from build123d import *

# Parameters (mm, degrees)
SKETCH1_W           = 7.2
SKETCH1_H           = 10.8
SKETCH1_R           = 1.75
BOSS_EXTRUDE3_DEPTH = 5
SKETCH2_W           = 50
SKETCH2_H           = 20
BOSS_EXTRUDE4_DEPTH = 5


with BuildPart() as part:
    # Sketch1 → Boss-Extrude3 (new body)
    with BuildSketch(Plane.XY):
        with Locations((10.9, 2.5)):
            Rectangle(SKETCH1_W, SKETCH1_H)
        Polygon((-20, 22.5), (-30, 11.319660113), (-30, -7.5), (-20, -22.5), (-4, -22.5), (6, -7.5), (30, -7.5), (30, 12.5), (6, 12.5), (-4, 22.5), align=None)
        with Locations((-17, -17.5)):
            Circle(SKETCH1_R, mode=Mode.SUBTRACT)
        with Locations((-7, -17.5)):
            Circle(SKETCH1_R, mode=Mode.SUBTRACT)
        with Locations((-25, 2.5)):
            Circle(SKETCH1_R, mode=Mode.SUBTRACT)
        Polygon((-3.5, 7.9), (7.3, 7.9), (14.5, 7.9), (14.5, -2.9), (7.3, -2.9), (-3.5, -2.9), align=None, mode=Mode.SUBTRACT)
    extrude(amount=BOSS_EXTRUDE3_DEPTH)

    # Sketch2 → Boss-Extrude4 (add)
    with BuildSketch(Plane(origin=(0, 0, 0), x_dir=(-1, 0, 0), z_dir=(0, 0, -1))):
        with Locations((-5, 2.5)):
            Rectangle(SKETCH2_W, SKETCH2_H)
    extrude(amount=-BOSS_EXTRUDE4_DEPTH)


solid = part.part
Source: CAD feature listing. Evaluate the final solid. Frame: model axes, mm. A direction names the side the tool comes from. Give positions to 0.01 mm unless a question says otherwise; leave off trailing zeros. Write each loop counter-clockwise with the first axis right and the second up, starting at its lowest first coordinate (ties: lowest second). Pieces come first, ordered by that corner, then holes. Notation, with made-up numbers: M 74,88.25 L 84,88.25 A11 ccw 84,97.25 Z; hole C 73,65 d3. An arc over 180 degrees is marked long. Return JSON: item names as keys, results as strings. Group by question number.
1) Cut plane C-C, the plane x = -25. Output: boundary loops of the cut face in (y, z).
2) Set-up query: faces 1 (the face through (-7, 0, 0)), 2 (the face through (18, -7.5, 2)), 3 (the face through (18, 12.5, 2)). Return all of +Z, -Z, +X, -X, +Y, -Y with unobstructed straight access to the full face (end or side cutting, diameter ignored); none if empty.
3) Cut plane D-D, the plane y = -17.5. Output: boundary loops of the cut face in (x, z).
4) Cut plane A-A, the plane y = 2.5. Output: boundary loops of the cut face in (x, z).
5) Cut plane B-B, the plane z = 2.1. Output: boundary loops of the cut face in (x, y), plus the area to 3 significant figures.
6) Material intervals for line 1 along Y through (x, z) = (-17, 2.15); line 2 along Y through (x, z) = (-8.5, 1.35); line 3 along X through (y, z) = (1, 1.4), sorted ascending. Write a range as [from, to].
7) Pull-direction query (Y, two-part tool) for faces 4 (the face through (-26.75, 2.58, 2.46)), 5 (the face through (-30, 2, 2)), 6 (the face through (-24.93, 16.99, 2.46)); classes: pulls with the +Y half, pulls with the -Y half, needs draft (parallel to the pull), parting line crosses it, or undercut.
8) Pin query (flat end, axial travel): P1, Ø3, axis at x = -17, y = -17.5, coming from the +Z side; P2, Ø2.5, axis at x = 20.5, z = 3, coming from the -Y side. Return the tip coordinate at first contact, or that it passes through.
Recorded:
{
 "1": {"outline": "M -15,0 L 0.75,0 L 0.75,5 L -15,5 Z; M 4.25,0 L 16.91,0 L 16.91,5 L 4.25,5 Z"},
 "2": {"face 1": "-Z, +X, -X, +Y, -Y", "face 2": "+Z, -Z, +X, -Y", "face 3": "+Z, -Z, +X, +Y"},
 "3": {"outline": "M -23.33,0 L -18.75,0 L -18.75,5 L -23.33,5 Z; M -15.25,0 L -8.75,0 L -8.75,5 L -15.25,5 Z; M -5.25,0 L -0.67,0 L -0.67,5 L -5.25,5 Z"},
 "4": {"outline": "M -30,0 L -26.75,0 L -26.75,5 L -30,5 Z; M -23.25,0 L 30,0 L 30,5 L -23.25,5 Z"},
 "5": {"outline": "M -30,-7.5 L -20,-22.5 L -4,-22.5 L 6,-7.5 L 30,-7.5 L 30,12.5 L 6,12.5 L -4,22.5 L -20,22.5 L -30,11.32 Z; hole C -25,2.5 d3.5; hole C -17,-17.5 d3.5; hole C -7,-17.5 d3.5", "area": "1,820 mm²"},
 "6": {"line 1": "y = [-22.5, -19.25], [-15.75, 22.5]", "line 2": "y = [-22.5, -18.4], [-16.6, 22.5]", "line 3": "x = [-30, -25.9], [-24.1, 30]"},
 "7": {"face 4": "undercut", "face 5": "needs draft", "face 6": "pulls with the +Y half"},
 "8": {"P1": "passes through", "P2": "stops at y = -7.5"}
}
